from build123d import *

# Parameters (mm, degrees)
F1_DEPTH = 3.175
F2_R     = 1.1938
F3_DEPTH = 2.54
F4_R     = 2.54
F5_DEPTH = 12.7


with BuildPart() as f1:
    # F0 (on Front) → F1 (new body)
    with BuildSketch(Plane.XZ):
        with BuildLine():
            Line((25.4, 6.35), (0, 6.35))
            ThreePointArc((0, 6.35), (-6.35, 0), (0, -6.35))
            Line((0, -6.35), (25.4, -6.35))
            ThreePointArc((25.4, -6.35), (31.75, 0), (25.4, 6.35))
        make_face()
    extrude(amount=F1_DEPTH)

    # F2 (on Front) → F3 (join)
    with BuildSketch(Plane.XZ):
        with Locations((10.16, 0)):
            Circle(F2_R)
        with Locations((26.67, 0)):
            Circle(F2_R)
    extrude(amount=-F3_DEPTH)

    # F4 (on Front) → F5 (join)
    with BuildSketch(Plane.XZ):
        with Locations((-1.4986, 0)):
            Circle(F4_R)
    extrude(amount=F5_DEPTH)


solid = f1.part
Geometry check sheet. Reference: the model listing, model coordinates, mm. A direction names the side the tool comes from. Round coordinates to 2 decimals unless told otherwise and drop trailing zeros. Write each loop counter-clockwise with the first axis right and the second up, starting at its lowest first coordinate (ties: lowest second). Pieces come first, ordered by that corner, then holes. Notation, with made-up numbers: (-10.5, 7) - (23.5, 7) arc R32 ccw to (23.5, 35) - close; hole circle Ø1 at (85.5, 28.25). An arc over 180 degrees is marked (long way). One line per item, written item: value.
1. Depth check by flat-ended pin: pin 1 Ø2 at (y, z) = (-1, -5) entering from -X; pin 2 Ø1.5 at (x, z) = (3, 4.5) entering from +Y; pin 3 Ø6 at (y, z) = (-7, 4.5) entering from +X. Enter the tip coordinate at first touch or a pass-through.
The answers:
pin 1: stops at x = -4.93
pin 2: stops at y = 0
pin 3: stops at x = 0.55
2. Cross-section at B-B on y = 0.75. Record the boundary of the cut face in (x, z), and give its area (3 significant figures).
The answers:
outline: circle Ø2.39 at (10.16, 0); circle Ø2.39 at (26.67, 0)
area: 8.95 mm^2
3. Cross-section at C-C on x = 10.16. Record the boundary of the cut face in (y, z) (3 decimals), and give its area (3 significant figures).
The answers:
outline: (-3.175, -6.35) - (0, -6.35) - (0, -1.194) - (2.54, -1.194) - (2.54, 1.194) - (0, 1.194) - (0, 6.35) - (-3.175, 6.35) - close
area: 46.4 mm^2
4. Set-up check for faces 1 (the face through (13, -2, 6.35)), 2 (the face through (25.79, 1.252, 0.807)): record each of +Z, -Z, +X, -X, +Y, -Y from which the full face is reachable in a straight line by a thin tool's end or side.
The answers:
face 1: +Z, +X, -X, +Y, -Y
face 2: +Y
5. Mould release check, pull along X, two halves, no side actions. Record for faces 3 (the face through (12, -3.175, 0)), 4 (the face through (0.924, -7.871, 0.763)), 5 (the face through (11.26, 1.25, -0.46)): released by +X, released by -X, zero draft, split by the parting line, or undercut.
The answers:
face 3: zero draft
face 4: split by the parting line
face 5: undercut
6. Cross-section at A-A on z = 0. Record the boundary of the cut face in (x, y) (3 decimals), and give its area (3 significant figures).
The answers:
outline: (-6.35, -3.175) - (-4.039, -3.175) - (-4.039, -12.7) - (1.041, -12.7) - (1.041, -3.175) - (31.75, -3.175) - (31.75, 0) - (27.864, 0) - (27.864, 2.54) - (25.476, 2.54) - (25.476, 0) - (11.354, 0) - (11.354, 2.54) - (8.966, 2.54) - (8.966, 0) - (-6.35, 0) - close
area: 181 mm^2
7. Cross-section at D-D on y = -2.25. Record the boundary of the cut face in (x, z).
The answers:
outline: (0, -6.35) - (25.4, -6.35) arc R6.35 ccw to (25.4, 6.35) - (0, 6.35) arc R6.35 ccw to start
8. Scan lines: L1, parallel to Y at x = 2.5, z = 5 (3 decimals); L2, parallel to X at y = -7.75, z = -1; L3, parallel to X at y = -3, z = 1.5. Record each from-to range of solid material in increasing order.
The answers:
L1: y = -3.175 to 0
L2: x = -3.83 to 0.84
L3: x = -6.17 to 31.57
